Can you work these out from the drawing? Everything is in mm from the part's minimum corner. A direction names the side the tool comes from. Coordinates: 2 decimals unless noted, no trailing zeros. Order: outer loops, then holes, each group sorted by start corner. A loop starts at its lowest first (then second) coordinate and runs counter-clockwise, first axis right, second up. Notation, with made-up numbers: (28, 70.5) -> (45, 70.5) arc R25 cw to (45, 96.5) -> close; hole circle Ø11 at (30.25, 25). An arc over 180 degrees is marked (long way). Return JSON: item names as keys, results as strings. Group by question number.
1) If we section it at B-B, the plane y = 5: Please give me the cut outline in (x, z).
2) If we section it at D-D, the plane z = 12.5: Please give me the cut outline in (x, y).
3) If I drill on probe 1 along Z at (x, y) = (2, 4.75); probe 2 along X at (y, z) = (6.5, 3.5); probe 3 along Y at (x, z) = (2.35, 1.25), over which ranges is the centre line in solid material (lowest first)? Write a range as from..to.
4) If we section it at A-A, the plane x = 35.65: Please give me the cut outline in (y, z), then the cut area to 4 significant figures.
5) If we section it at C-C, the plane x = 13.5: Please give me the cut outline in (y, z).
6) For the marked faces 1, 2 and 3, which set-ups out of +Z, -Z, +X, -X, +Y, -Y let a thin tool reach every point of the face, with its end or its side?
7) For pin 1 (5 mm diameter, centred on x = 28.5, z = 4, fed in from +Y) (3 decimals); pin 2 (7 mm diameter, centred on x = 1.5, y = 12.5, fed in from +Z); pin 3 (6 mm diameter, centred on x = 33.5, y = 16.5, fed in from -Z); pin 4 (6 mm diameter, centred on x = 22, z = 1.5, fed in from -Y), each with a flat end and sliding along its axis, tell me the tip position at first contact or that it passes through.
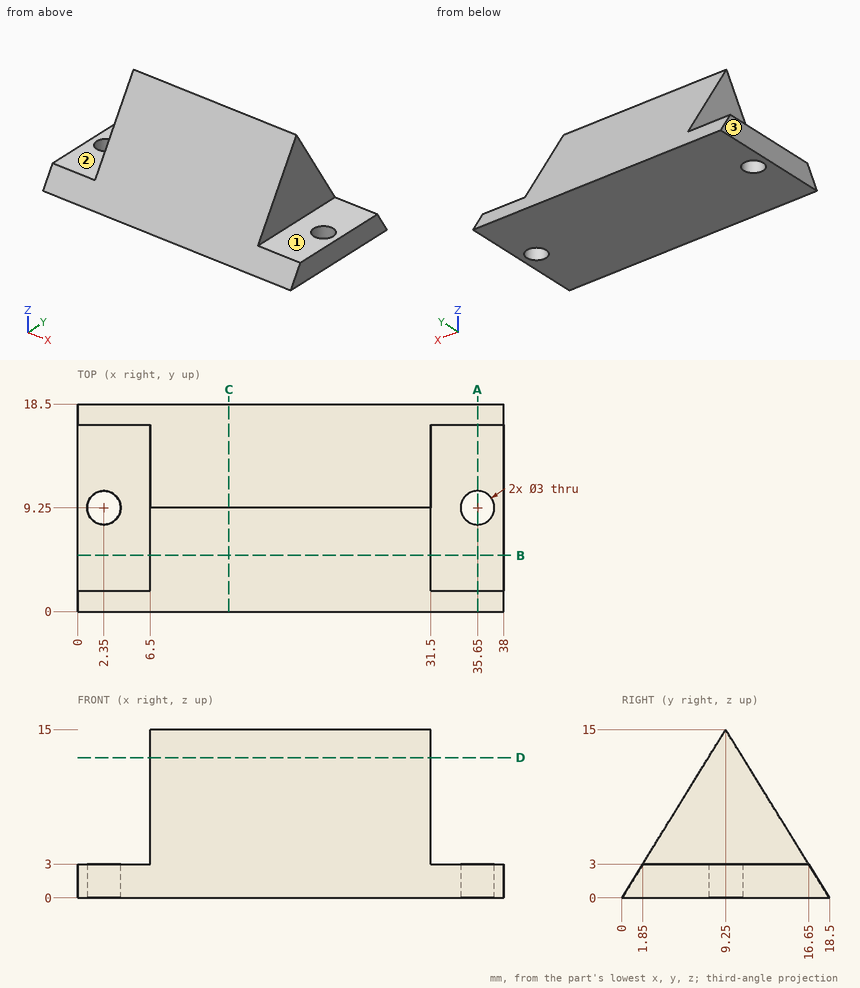
Result sheet:
{
 "1": {"outline": "(0, 0) -> (38, 0) -> (38, 3) -> (31.5, 3) -> (31.5, 8.11) -> (6.5, 8.11) -> (6.5, 3) -> (0, 3) -> close"},
 "2": {"outline": "(6.5, 7.71) -> (31.5, 7.71) -> (31.5, 10.79) -> (6.5, 10.79) -> close"},
 "3": {"probe 1": "z = 0..3", "probe 2": "x = 6.5..31.5", "probe 3": "y = 0.77..7.75, 10.75..17.73"},
 "4": {"outline": "(0, 0) -> (7.75, 0) -> (7.75, 3) -> (1.85, 3) -> close; (10.75, 0) -> (18.5, 0) -> (16.65, 3) -> (10.75, 3) -> close", "area": "40.95 mm2"},
 "5": {"outline": "(0, 0) -> (18.5, 0) -> (9.25, 15) -> close"},
 "6": {"face 1": "+Z, +X, +Y, -Y", "face 2": "+Z, -X, +Y, -Y", "face 3": "+Z, -Z, -X, +Y, -Y"},
 "7": {"pin 1": "stops at y = 17.575", "pin 2": "stops at z = 3", "pin 3": "stops at z = 0", "pin 4": "stops at y = 0"}
}
